Can you work these out from the model? Positions are in its coordinate system, mm. A direction names the side the tool comes from. Round coordinates to 2 decimals unless told otherwise and drop trailing zeros. Loops run counter-clockwise (first coordinate to the right, second up) from the corner with the lowest first, then second, coordinate; pieces in that order, holes last.
```python
from build123d import *

# Parameters (mm, degrees)
F0_W     = 15
F0_H     = 15
F1_DEPTH = 2
F2_W     = 13
F2_H     = 13
F3_DEPTH = 10
F5_DEPTH = 12
F7_DEPTH = 5


# Not quite as in the source:
# - a feature names something its author has since deleted; it is built from what else it names


with BuildPart() as f1:
    # F0 (on Front) → F1 (new body)
    with BuildSketch(Plane.XZ):
        Rectangle(F0_W, F0_H)
    extrude(amount=F1_DEPTH)

    # F2 (on face) → F3 (join)
    with BuildSketch(Plane.XZ.offset(2)):
        Rectangle(F2_W, F2_H)
    extrude(amount=F3_DEPTH)

    # F4 (on face) → F5 (cut, through all)
    with BuildSketch(Plane(origin=(0, 0, 0), x_dir=(-1, 0, 0), z_dir=(0, 1, 0))):
        Polygon((1.5, -0.8660254038), (1.5, 0.8660254038), (0, 1.7320508076), (-1.5, 0.8660254038), (-1.5, -0.8660254038), (0, -1.7320508076), align=None)
    extrude(amount=-F5_DEPTH, mode=Mode.SUBTRACT)

    # F6 (on face) → F7 (cut)
    with BuildSketch(Plane.XZ.offset(12)):
        Polygon((-2.8, 1.6165807537), (-2.8, -1.6165807537), (0, -3.2331615075), (2.8, -1.6165807537), (2.8, 1.6165807537), (0, 3.2331615075), align=None)
        Polygon((1.5, 0.8660254038), (1.5, -0.8660254038), (0, -1.7320508076), (-1.5, -0.8660254038), (-1.5, 0.8660254038), (0, 1.7320508076), align=None, mode=Mode.SUBTRACT)
    extrude(amount=-F7_DEPTH, mode=Mode.SUBTRACT)


solid = f1.part
```
(1) Which directions (+Z, -Z, +X, -X, +Y, -Y) give clear straight access to the entire face, cutting with the end or side of a thin tool? Please do faces 1 (the flat face through (-6.5, -7, 0)), 2 (the flat face through (0.76, -3.451, -1.293)), 3 (the flat face through (1.42, -9.535, 2.414)).
(2) Suppose I cut it at A-A (y = -1.25). Write out the boundary of the cut face in (x, z), then the cut area to 3 significant figures.
(3) Suppose I cut it at C-C (x = -6.25). Write out the boundary of the cut face in (y, z).
(4) We'd pull the mould along Z, two halves only. Please class faces 4 (the flat face through (0, -7, -6.5)), 5 (the flat face through (-2.8, -10, 0)), 6 (the flat face through (-3, -12, 0)): released by +Z, released by -Z, zero draft, split by the parting line, or undercut.
(5) For pin 1 (0.9 mm diameter, centred on y = -4.5, z = -0.5, fed in from -X); pin 2 (2.5 mm diameter, centred on y = -10.5, z = 0, fed in from +X); pin 3 (5 mm diameter, centred on x = 2, y = -5, fed in from -Z), each with a flat end and sliding along its axis, tell me the tip position at first contact or that it passes through.
(6) If I drill on line 1 (X direction, y = -5.5, z = -0.5); line 2 (X direction, y = -11.5, z = 0.75); line 3 (X direction, y = -6.25, z = -4), over which ranges is the centre line in solid material (lowest first)?
(7) Suppose I cut it at B-B (z = 4.5). Write out the boundary of the cut face in (x, y), then the cut area to 3 significant figures.
(8) Suppose I cut it at D-D (y = -9). Write out the boundary of the cut face in (x, z), then the cut area to 3 significant figures.
Check result:
1. face 1: +Z, -Z, -X, -Y
1. face 2: +Y, -Y
1. face 3: -Y
2. outline: (-7.5, -7.5) - (7.5, -7.5) - (7.5, 7.5) - (-7.5, 7.5) - close; hole (-1.5, -0.87) - (0, -1.73) - (1.5, -0.87) - (1.5, 0.87) - (0, 1.73) - (-1.5, 0.87) - close
2. area: 217 mm2
3. outline: (-12, -6.5) - (-2, -6.5) - (-2, -7.5) - (0, -7.5) - (0, 7.5) - (-2, 7.5) - (-2, 6.5) - (-12, 6.5) - close
4. face 4: released by -Z
4. face 5: undercut
4. face 6: zero draft
5. pin 1: stops at x = -6.5
5. pin 2: stops at x = 6.5
5. pin 3: stops at z = -6.5
6. line 1: x = -6.5 to -1.5, 1.5 to 6.5
6. line 2: x = -6.5 to -2.8, 2.8 to 6.5
6. line 3: x = -6.5 to 6.5
7. outline: (-7.5, -2) - (-6.5, -2) - (-6.5, -12) - (6.5, -12) - (6.5, -2) - (7.5, -2) - (7.5, 0) - (-7.5, 0) - close
7. area: 160 mm2
8. outline: (-6.5, -6.5) - (6.5, -6.5) - (6.5, 6.5) - (-6.5, 6.5) - close; hole (-2.8, -1.62) - (0, -3.23) - (2.8, -1.62) - (2.8, 1.62) - (0, 3.23) - (-2.8, 1.62) - close
8. area: 142 mm2
